```python
from build123d import *

# Parameters (mm, degrees)
PAD024_DEPTH         = 2
SKETCH118_W          = 5
SKETCH118_H          = 1.8
POCKET028_DEPTH      = 23.716818
POCKET028_DEPTH_BACK = 25.616818


with BuildPart() as part:
    # Sketch119 → Pad024 (new body, symmetric)
    with BuildSketch(Plane.XZ):
        with BuildLine():
            Line((0, 1.9), (3.2, 1.9))
            ThreePointArc((3.677897, 1.547019), (3.497061, 1.802188), (3.2, 1.9))
            Line((4, 0.5), (3.677897, 1.547019))
            Line((4, 0.5), (5.5, 0.5))
            Line((5.5, 0.5), (5.5, 0))
            Line((5.5, 0), (4, 0))
            ThreePointArc((3.522103, 0.352981), (3.702939, 0.097812), (4, 0))
            Line((3.2, 1.4), (3.522103, 0.352981))
            Line((3.2, 1.4), (0, 1.4))
            Line((0, 1.4), (0, 1.9))
        make_face()
    pad024 = extrude(amount=PAD024_DEPTH, both=True)

    # Mirrored020: Pad024 across YZ
    add(pad024.mirror(Plane.YZ))

    # Sketch118 → Pocket028 (cut, two sides)
    with BuildSketch(Plane.XY) as pocket028_sk:
        with Locations((3.5, 0)):
            Rectangle(SKETCH118_W, SKETCH118_H)
    pocket028 = extrude(amount=-POCKET028_DEPTH, mode=Mode.SUBTRACT) + extrude(pocket028_sk.sketch, amount=POCKET028_DEPTH_BACK, mode=Mode.SUBTRACT)

    # Mirrored003: Pocket028 across YZ
    add(pocket028.mirror(Plane.YZ), mode=Mode.SUBTRACT)


with BuildPart() as part_1:
    # Body033 placement: moved
    add(part.part.moved(Location((0, 12.65, 0))))


solid = part_1.part
```
Verification items for the finished model (mm, model axes). A direction names the side the tool comes from. Round coordinates to 2 decimals unless told otherwise and drop trailing zeros. Order: outer loops, then holes, each group sorted by start corner. A loop starts at its lowest first (then second) coordinate and runs counter-clockwise, first axis right, second up.
1) Depth check by flat-ended pin: pin 1 (0.6 mm diameter, centred on x = 3, z = 0.5, fed in from -Y); pin 2 (0.5 mm diameter, centred on x = 5, y = 11, fed in from +Z); pin 3 (1 mm diameter, centred on x = -4, z = 1, fed in from -Y). Enter the tip coordinate at first touch or a pass-through.
Geometry says:
pin 1: passes through
pin 2: stops at z = 0.5
pin 3: stops at y = 10.65
2) Material ranges on line 1 (Y direction, x = 3.75, z = 1.05); line 2 (Z direction, x = -1.25, y = 10.95); line 3 (Z direction, x = -4.25, y = 13.8), recorded low to high.
Geometry says:
line 1: y = 10.65 to 11.75, 13.55 to 14.65
line 2: z = 1.4 to 1.9
line 3: z = 0 to 0.5
3) Tool access check on faces 3 (the flat face through (3.41, 11.75, 1.23)), 4 (the flat face through (-3.36, 11.19, 0.88)), 5 (the flat face through (5, 11, 0.5)). Record the directions out of +Z, -Z, +X, -X, +Y, -Y that give a thin tool (end or side, any length) a straight path to the whole face; none if there is none.
Geometry says:
face 3: +Z, -Z, +X
face 4: -Z, +Y, -Y
face 5: +Z, +X, +Y, -Y
4) Draft check along Y on faces 1 (the flat face through (5, 14, 0.5)), 2 (the flat face through (-3.6, 11.75, 1.1)). Enter one of: +Y half, -Y half, draft (parallel to the pull), parting line (faces both ways), or undercut.
Geometry says:
face 1: draft
face 2: undercut
5) Cross-section at A-A, the plane x = -4.75. Record the cut outline in (y, z).
Geometry says:
outline: (10.65, 0) - (11.75, 0) - (11.75, 0.5) - (10.65, 0.5) - close; (13.55, 0) - (14.65, 0) - (14.65, 0.5) - (13.55, 0.5) - close
6) Cross-section at D-D, the plane z = 1.75. Record the cut outline in (x, y).
Geometry says:
outline: (-3.56, 10.65) - (3.56, 10.65) - (3.56, 11.75) - (1, 11.75) - (1, 13.55) - (3.56, 13.55) - (3.56, 14.65) - (-3.56, 14.65) - (-3.56, 13.55) - (-1, 13.55) - (-1, 11.75) - (-3.56, 11.75) - close
7) Cross-section at B-B, the plane z = 1.3. Record the cut outline in (x, y), plus the area to 3 significant figures.
Geometry says:
outline: (-3.75, 10.65) - (-3.23, 10.65) - (-3.23, 11.75) - (-3.75, 11.75) - close; (-3.75, 13.55) - (-3.23, 13.55) - (-3.23, 14.65) - (-3.75, 14.65) - close; (3.23, 10.65) - (3.75, 10.65) - (3.75, 11.75) - (3.23, 11.75) - close; (3.23, 13.55) - (3.75, 13.55) - (3.75, 14.65) - (3.23, 14.65) - close
area: 2.30 mm2
8) Cross-section at C-C, the plane y = 14.15. Record the cut outline in (x, z).
Geometry says:
outline: (-5.5, 0) - (-4, 0) arc R0.5 ccw to (-3.52, 0.35) - (-3.2, 1.4) - (3.2, 1.4) - (3.52, 0.35) arc R0.5 ccw to (4, 0) - (5.5, 0) - (5.5, 0.5) - (4, 0.5) - (3.68, 1.55) arc R0.5 ccw to (3.2, 1.9) - (-3.2, 1.9) arc R0.5 ccw to (-3.68, 1.55) - (-4, 0.5) - (-5.5, 0.5) - close
